from build123d import *

# Parameters (mm, degrees)
BOSS_EXTRUDE1_DEPTH = 3.5
SKETCH2_R           = 1.5
CUT_EXTRUDE1_DEPTH  = 26.734218465


with BuildPart() as part:
    # Sketch1 → Boss-Extrude1 (new body)
    with BuildSketch(Plane(origin=(0, 0, 0), x_dir=(1, 0, 0), z_dir=(0, 1, 0))):
        with BuildLine():
            Line((-18.607695155, -5), (18.607695155, -5))
            Line((18.607695155, -5), (21, -5))
            ThreePointArc((21, -5), (24.863703305, -2.03527618), (23, 2.464101615))
            Line((23, 2.464101615), (18.607695155, 5))
            Line((18.607695155, 5), (-18.607695155, 5))
            Line((-18.607695155, 5), (-23, 2.464101615))
            ThreePointArc((-23, 2.464101615), (-24.863703305, -2.03527618), (-21, -5))
            Line((-21, -5), (-18.607695155, -5))
        make_face()
    extrude(amount=BOSS_EXTRUDE1_DEPTH)

    # Sketch2 → Cut-Extrude1 (cut, through all)
    with BuildSketch(Plane(origin=(0, 3.5, 0), x_dir=(1, 0, 0), z_dir=(0, 1, 0))):
        with Locations(Location((-21, -1, 0), (0, 0, 270))):
            Circle(SKETCH2_R)
        with Locations(Location((21, -1, 0), (0, 0, 270))):
            Circle(SKETCH2_R)
    extrude(amount=-CUT_EXTRUDE1_DEPTH, mode=Mode.SUBTRACT)


solid = part.part
Could you check a few things on this model? Use its own coordinates, in mm. Coordinates: 2 decimals unless noted, no trailing zeros. Order: outer loops, then holes, each group sorted by start corner. A loop starts at its lowest first (then second) coordinate and runs counter-clockwise, first axis right, second up. Notation, with made-up numbers: (81.25, 57) -> (127.25, 57) arc R9 ccw to (127.25, 65) -> close; hole circle Ø4 at (-17.5, 20). An arc over 180 degrees is marked (long way). One line per item, written item: value. Start each with the question number.
1) Imagine slicing it at B-B on y = 2.7. List the corners of the cut face in (x, z) for me, plus the area to 3 significant figures.
2) Imagine slicing it at A-A on z = 1. List the corners of the cut face in (x, y) for me, plus the area to 3 significant figures.
3) We'd pull the mould along X, two halves only. Please class faces 1 (the cylindrical face through (-19.735, 1.774, 1.806)), 2 (the cylindrical face through (24.844, 1.726, 2.106)), 3 (the flat face through (0, 0, 0)), 4 (the cylindrical face through (-24.882, 1.726, 1.964)): +X half, -X half, draft (parallel to the pull), parting line (faces both ways), or undercut.
4) I'm going to push a flat-ended pin straight in: pin 1 (1.5 mm diameter, centred on y = 2.5, z = -1.5, fed in from +X). Where does the tip first touch, or does it pass through?
5) If I drill on L1, parallel to X at y = 2, z = 1; L2, parallel to X at y = 2.9, z = 0.5; L3, parallel to X at y = 1.3, z = -2.25, over which ranges is the centre line in solid material (lowest first)? Write a range as [from, to].
6) Imagine slicing it at C-C on z = -1.25. List the corners of the cut face in (x, y) for me, plus the area to 3 significant figures.
Answer list:
1. outline: (-23, -2.46) -> (-18.61, -5) -> (18.61, -5) -> (23, -2.46) arc R4 ccw to (21, 5) -> (-21, 5) arc R4 ccw to start; hole circle Ø3 at (-21, 1); hole circle Ø3 at (21, 1)
1. area: 454 mm2
2. outline: (-25, 0) -> (-22.5, 0) -> (-22.5, 3.5) -> (-25, 3.5) -> close; (-19.5, 0) -> (19.5, 0) -> (19.5, 3.5) -> (-19.5, 3.5) -> close; (22.5, 0) -> (25, 0) -> (25, 3.5) -> (22.5, 3.5) -> close
2. area: 154 mm2
3. face 1: undercut
3. face 2: +X half
3. face 3: draft
3. face 4: -X half
4. pin 1: stops at x = 24.6
5. L1: x = [-25, -22.5], [-19.5, 19.5], [22.5, 25]
5. L2: x = [-24.97, -22.41], [-19.59, 19.59], [22.41, 24.97]
5. L3: x = [-23.33, 23.33]
6. outline: (-24.31, 0) -> (24.31, 0) -> (24.31, 3.5) -> (-24.31, 3.5) -> close
6. area: 170 mm2
